from build123d import *

# Parameters (mm, degrees)
SKETCH1_W           = 55.5
SKETCH1_H           = 21.7
BOSS_EXTRUDE1_DEPTH = 15
SKETCH3_R           = 1.65
CUT_EXTRUDE1_DEPTH  = 16
FILLET1_R           = 1


with BuildPart() as part:
    # Sketch1 → Boss-Extrude1 (new body)
    with BuildSketch(Plane.XY):
        Rectangle(SKETCH1_W, SKETCH1_H)
    extrude(amount=BOSS_EXTRUDE1_DEPTH)

    # Sketch3 → Cut-Extrude1 (cut, through all)
    with BuildSketch(Plane.XY.offset(15)):
        with Locations((-20.25, 4.85)):
            Circle(SKETCH3_R)
        with Locations((-20.25, -4.85)):
            Circle(SKETCH3_R)
        with Locations((20.25, -4.85)):
            Circle(SKETCH3_R)
        with Locations((20.25, 4.85)):
            Circle(SKETCH3_R)
    extrude(amount=-CUT_EXTRUDE1_DEPTH, mode=Mode.SUBTRACT)

    # Fillet1
    fillet1_edges = [part.edges().sort_by_distance(p)[0] for p in [
        (0, -10.85, 0),
        (0, 10.85, 0),
    ]]
    fillet(fillet1_edges, radius=FILLET1_R)


solid = part.part
Could you check a few things on this model? Use its own coordinates, in mm. Coordinates: 2 decimals unless noted, no trailing zeros. Order: outer loops, then holes, each group sorted by start corner. A loop starts at its lowest first (then second) coordinate and runs counter-clockwise, first axis right, second up. Notation, with made-up numbers: (37.25, 63) -> (62.25, 63) arc R19 cw to (62.25, 93) -> close; hole circle Ø1 at (34.25, 49). An arc over 180 degrees is marked (long way). One line per item, written item: value. Start each with the question number.
1) Imagine slicing it at A-A on z = 6.25. List the corners of the cut face in (x, y) for me, plus the area to 3 significant figures.
2) Imagine slicing it at B-B on x = 20.25. List the corners of the cut face in (y, z) for me, plus the area to 3 significant figures.
3) Imagine slicing it at D-D on x = -21. List the corners of the cut face in (y, z) for me, plus the area to 3 significant figures.
4) If I drill on L1, parallel to Y at x = -20.25, z = 10.75; L2, parallel to X at y = -4.75, z = 12.5; L3, parallel to X at y = 4, z = 6.5, over which ranges is the centre line in solid material (lowest first)? Write a range as [from, to].
5) We'd pull the mould along Y, two halves only. Please class faces 1 (the flat face through (0, 10.85, 8)), 2 (the cylindrical face through (-21.9, 4.9, 7.6)), 3 (the flat face through (0, -10.85, 8)): +Y half, -Y half, draft (parallel to the pull), parting line (faces both ways), or undercut.
6) Imagine slicing it at C-C on y = -4.85. List the corners of the cut face in (x, z) for me.
Answer list:
1. outline: (-27.75, -10.85) -> (27.75, -10.85) -> (27.75, 10.85) -> (-27.75, 10.85) -> close; hole circle Ø3.3 at (-20.25, -4.85); hole circle Ø3.3 at (-20.25, 4.85); hole circle Ø3.3 at (20.25, -4.85); hole circle Ø3.3 at (20.25, 4.85)
1. area: 1,170 mm2
2. outline: (-10.85, 1) arc R1 ccw to (-9.85, 0) -> (-6.5, 0) -> (-6.5, 15) -> (-10.85, 15) -> close; (-3.2, 0) -> (3.2, 0) -> (3.2, 15) -> (-3.2, 15) -> close; (6.5, 0) -> (9.85, 0) arc R1 ccw to (10.85, 1) -> (10.85, 15) -> (6.5, 15) -> close
2. area: 226 mm2
3. outline: (-10.85, 1) arc R1 ccw to (-9.85, 0) -> (-6.32, 0) -> (-6.32, 15) -> (-10.85, 15) -> close; (-3.38, 0) -> (3.38, 0) -> (3.38, 15) -> (-3.38, 15) -> close; (6.32, 0) -> (9.85, 0) arc R1 ccw to (10.85, 1) -> (10.85, 15) -> (6.32, 15) -> close
3. area: 237 mm2
4. L1: y = [-10.85, -6.5], [-3.2, 3.2], [6.5, 10.85]
4. L2: x = [-27.75, -21.9], [-18.6, 18.6], [21.9, 27.75]
4. L3: x = [-27.75, -21.66], [-18.84, 18.84], [21.66, 27.75]
5. face 1: +Y half
5. face 2: undercut
5. face 3: -Y half
6. outline: (-27.75, 0) -> (-21.9, 0) -> (-21.9, 15) -> (-27.75, 15) -> close; (-18.6, 0) -> (18.6, 0) -> (18.6, 15) -> (-18.6, 15) -> close; (21.9, 0) -> (27.75, 0) -> (27.75, 15) -> (21.9, 15) -> close
